Check sheet for the drawn part. Datum: minimum x, y, z corner. Units: mm. Coordinates: 2 decimals unless noted, no trailing zeros. Order: outer loops, then holes, each group sorted by start corner. A loop starts at its lowest first (then second) coordinate and runs counter-clockwise, first axis right, second up. Notation, with made-up numbers: M 69.5,25.25 L 97.5,25.25 A26 ccw 97.5,57.25 Z; hole C -3.75,64 d5. An arc over 180 degrees is marked long. Return JSON: item names as keys, results as strings. Group by question number.
Q1. Thickness scan on probe 1 along X at (y, z) = (0.3, 2.3); probe 2 along X at (y, z) = (4.55, 3.4); probe 3 along Z at (x, y) = (12.5, 2.2). Record the ranges inside material, lowest first.
Q2. Section check C-C, the plane x = 7.5. Enter the section's corners in (y, z), then the cut area to 3 significant figures.
Q3. Mould release check, pull along Y, two halves, no side actions. Record for the marked faces 1, 2 and 3: pulls with the +Y half, pulls with the -Y half, needs draft (parallel to the pull), parting line crosses it, or undercut.
Q4. Go/stop test with a flat-tipped pin: pin 1 Ø2 at (x, y) = (7.5, 2.5) entering from -Z. Record where the tip stops, or that it passes through.
Q5. Section check A-A, the plane y = 2.5. Enter the section's corners in (x, z), then the cut area to 3 significant figures.
Q6. Section check B-B, the plane z = 2.5. Enter the section's corners in (x, y).
Q7. Section check D-D, the plane y = 0.7. Enter the section's corners in (x, z), then the cut area to 3 significant figures.
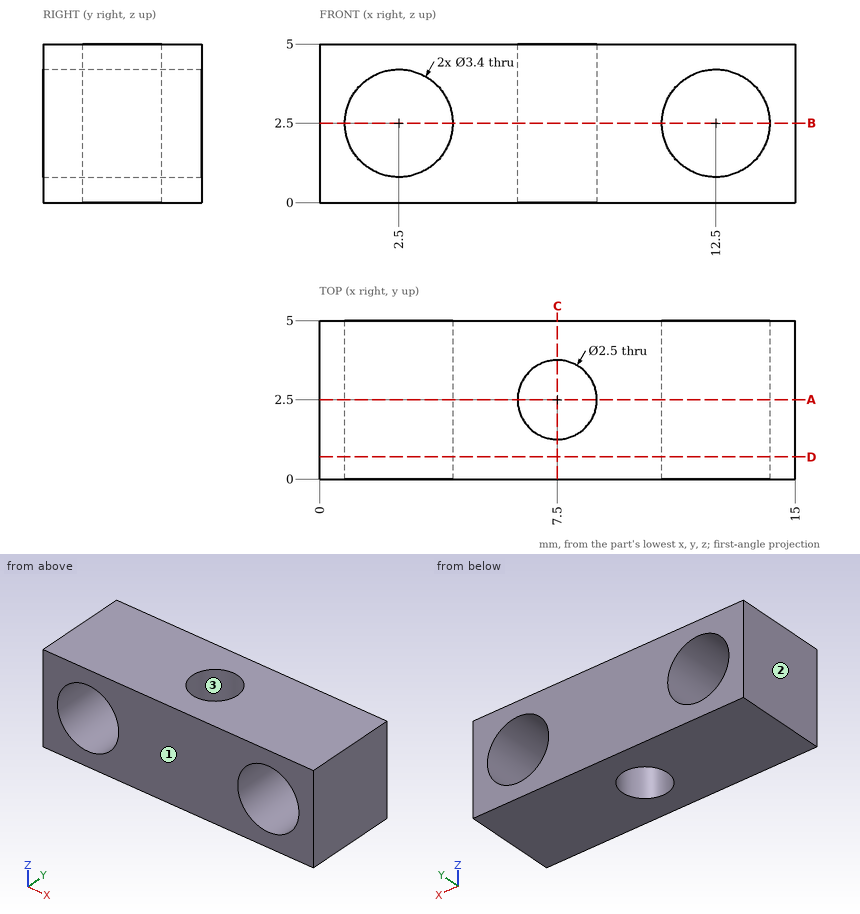
Numbers:
{
 "1": {"probe 1": "x = 0 to 0.81, 4.19 to 10.81, 14.19 to 15", "probe 2": "x = 0 to 1.06, 3.94 to 11.06, 13.94 to 15", "probe 3": "z = 0 to 0.8, 4.2 to 5"},
 "2": {"outline": "M 0,0 L 1.25,0 L 1.25,5 L 0,5 Z; M 3.75,0 L 5,0 L 5,5 L 3.75,5 Z", "area": "12.5 mm2"},
 "3": {"face 1": "pulls with the -Y half", "face 2": "needs draft", "face 3": "undercut"},
 "4": {"pin 1": "passes through"},
 "5": {"outline": "M 0,0 L 6.25,0 L 6.25,5 L 0,5 Z; M 8.75,0 L 15,0 L 15,5 L 8.75,5 Z; hole C 2.5,2.5 d3.4; hole C 12.5,2.5 d3.4", "area": "44.3 mm2"},
 "6": {"outline": "M 0,0 L 0.8,0 L 0.8,5 L 0,5 Z; M 4.2,0 L 10.8,0 L 10.8,5 L 4.2,5 Z; M 14.2,0 L 15,0 L 15,5 L 14.2,5 Z; hole C 7.5,2.5 d2.5"},
 "7": {"outline": "M 0,0 L 15,0 L 15,5 L 0,5 Z; hole C 2.5,2.5 d3.4; hole C 12.5,2.5 d3.4", "area": "56.8 mm2"}
}
